```python
from build123d import *

# Parameters (mm, degrees)
SKETCH1_W           = 40
SKETCH1_H           = 12.5
BOSS_EXTRUDE1_DEPTH = 4
SKETCH2_R           = 1.65
CUT_EXTRUDE1_DEPTH  = 43.09809972
SKETCH3_W           = 11
SKETCH3_H           = 2.9
CUT_EXTRUDE2_DEPTH  = 1.5
FILLET1_R           = 3


with BuildPart() as part:
    # Sketch1 → Boss-Extrude1 (new body)
    with BuildSketch(Plane(origin=(0, 0, 0), x_dir=(1, 0, 0), z_dir=(0, 1, 0))):
        with Locations((20, -6.25)):
            Rectangle(SKETCH1_W, SKETCH1_H)
    extrude(amount=BOSS_EXTRUDE1_DEPTH)

    # Sketch2 → Cut-Extrude1 (cut, through all)
    with BuildSketch(Plane(origin=(0, 4, 0), x_dir=(1, 0, 0), z_dir=(0, 1, 0))):
        with Locations(Location((4.85, -6.25, 0), (0, 0, 270))):
            Circle(SKETCH2_R)
        with Locations(Location((13, -6.25, 0), (0, 0, 270))):
            Circle(SKETCH2_R)
        with Locations(Location((27, -6.25, 0), (0, 0, 270))):
            Circle(SKETCH2_R)
        with Locations(Location((35.15, -6.25, 0), (0, 0, 270))):
            Circle(SKETCH2_R)
    extrude(amount=-CUT_EXTRUDE1_DEPTH, mode=Mode.SUBTRACT)

    # Sketch3 → Cut-Extrude2 (cut)
    with BuildSketch(Plane(origin=(0, 4, 0), x_dir=(1, 0, 0), z_dir=(0, 1, 0))):
        with Locations((20, -3.25)):
            Rectangle(SKETCH3_W, SKETCH3_H)
        with Locations((20, -9.05)):
            Rectangle(SKETCH3_W, SKETCH3_H)
    extrude(amount=-CUT_EXTRUDE2_DEPTH, mode=Mode.SUBTRACT)

    # Fillet1
    fillet1_edges = [part.edges().sort_by_distance(p)[0] for p in [
        (0, 2, 0),
        (40, 2, 0),
        (40, 2, 12.5),
        (0, 2, 12.5),
    ]]
    fillet(fillet1_edges, radius=FILLET1_R)


solid = part.part
```
Design review of the part built by this model. Coordinates are the model's own, in mm. A direction names the side the tool comes from. Coordinates: 2 decimals unless noted, no trailing zeros. Order: outer loops, then holes, each group sorted by start corner. A loop starts at its lowest first (then second) coordinate and runs counter-clockwise, first axis right, second up. Notation, with made-up numbers: (-3.5, 54) -> (4.5, 54) arc R32 cw to (4.5, 89) -> close; hole circle Ø8 at (59.25, 20). An arc over 180 degrees is marked (long way). One line per item, written item: value. Start each with the question number.
Q1. Tool access review of faces 5 (the cylindrical face through (36.786, 2.028, 6.035)), 6 (the flat face through (14.5, 3, 3)): name each direction out of +Z, -Z, +X, -X, +Y, -Y from which nothing blocks a thin tool from reaching the whole face with its end or side.
Q2. Take a section at A-A, the plane x = 13. State the section outline as (y, z) points, then the cut area to 3 significant figures.
Q3. Take a section at D-D, the plane y = 3.55. State the section outline as (x, z) points, then the cut area to 3 significant figures.
Q4. Insertion check: pin 1 Ø6 at (x, z) = (19.5, 4.5) entering from +Y; pin 2 Ø2.5 at (x, z) = (35.15, 6.25) entering from +Y; pin 3 Ø0.9 at (x, z) = (18.5, 9) entering from +Y. Each pin has a flat end and moves straight along its axis. Give the tip position at first contact, or say it passes through.
Q5. Mouldability with a two-part tool opening along Z and no side actions: class faces 1 (the flat face through (20, 3, 4.7)), 2 (the cylindrical face through (0.86, 2.03, 0.9)), 3 (the flat face through (40, 2, 6)), 4 (the cylindrical face through (39.1, 2.03, 11.64)) as pulls with the +Z half, pulls with the -Z half, needs draft (parallel to the pull), parting line crosses it, or undercut.
Q6. Take a section at B-B, the plane y = 1.4. State the section outline as (x, z) points.
Q7. For probe 1 along X at (y, z) = (2.05, 6.25); probe 2 along Z at (x, y) = (20.5, 3.85); probe 3 along X at (y, z) = (3.15, 8.5), list the stretches that pass through material, from the lowest coordinate up.
Q8. Take a section at C-C, the plane z = 6.25. State the section outline as (x, y) points.
Values follow:
1. face 5: +Y, -Y
1. face 6: +Y
2. outline: (0, 0) -> (4, 0) -> (4, 4.6) -> (0, 4.6) -> close; (0, 7.9) -> (4, 7.9) -> (4, 12.5) -> (0, 12.5) -> close
2. area: 36.8 mm2
3. outline: (0, 3) arc R3 ccw to (3, 0) -> (37, 0) arc R3 ccw to (40, 3) -> (40, 9.5) arc R3 ccw to (37, 12.5) -> (3, 12.5) arc R3 ccw to (0, 9.5) -> close; hole circle Ø3.3 at (4.85, 6.25); hole circle Ø3.3 at (13, 6.25); hole (14.5, 1.8) -> (25.5, 1.8) -> (25.5, 4.7) -> (14.5, 4.7) -> close; hole (14.5, 7.6) -> (25.5, 7.6) -> (25.5, 10.5) -> (14.5, 10.5) -> close; hole circle Ø3.3 at (27, 6.25); hole circle Ø3.3 at (35.15, 6.25)
3. area: 394 mm2
4. pin 1: stops at y = 4
4. pin 2: passes through
4. pin 3: stops at y = 2.5
5. face 1: undercut
5. face 2: pulls with the -Z half
5. face 3: needs draft
5. face 4: pulls with the +Z half
6. outline: (0, 3) arc R3 ccw to (3, 0) -> (37, 0) arc R3 ccw to (40, 3) -> (40, 9.5) arc R3 ccw to (37, 12.5) -> (3, 12.5) arc R3 ccw to (0, 9.5) -> close; hole circle Ø3.3 at (4.85, 6.25); hole circle Ø3.3 at (13, 6.25); hole circle Ø3.3 at (27, 6.25); hole circle Ø3.3 at (35.15, 6.25)
7. probe 1: x = 0 to 3.2, 6.5 to 11.35, 14.65 to 25.35, 28.65 to 33.5, 36.8 to 40
7. probe 2: z = 0 to 1.8, 4.7 to 7.6, 10.5 to 12.5
7. probe 3: x = 0 to 14.5, 25.5 to 40
8. outline: (0, 0) -> (3.2, 0) -> (3.2, 4) -> (0, 4) -> close; (6.5, 0) -> (11.35, 0) -> (11.35, 4) -> (6.5, 4) -> close; (14.65, 0) -> (25.35, 0) -> (25.35, 4) -> (14.65, 4) -> close; (28.65, 0) -> (33.5, 0) -> (33.5, 4) -> (28.65, 4) -> close; (36.8, 0) -> (40, 0) -> (40, 4) -> (36.8, 4) -> close
